```python
from build123d import *

# Parameters (mm, degrees)
F0_R     = 7
F1_DEPTH = 1
F2_R     = 5.5
F3_DEPTH = 8
F4_R     = 7
F5_DEPTH = 7
F6_R     = 0.6
F7_DEPTH = 8
F8_R     = 2.5
F9_DEPTH = 16.001
F10_SIZE = 0.25


with BuildPart() as f1:
    # F0 (on Front) → F1 (new body)
    with BuildSketch(Plane.XZ):
        Circle(F0_R)
    extrude(amount=F1_DEPTH)

    # F2 (on face) → F3 (join)
    with BuildSketch(Plane.XZ.offset(1)):
        Circle(F2_R)
    extrude(amount=F3_DEPTH)

    # F4 (on face) → F5 (join)
    with BuildSketch(Plane.XZ.offset(9)):
        Circle(F4_R)
    extrude(amount=F5_DEPTH)

    # F6 (on face) → F7 (cut, through all)
    with BuildSketch(Plane.XZ.offset(1)):
        with Locations((0, 5.5)):
            Circle(F6_R)
        with Locations((-2.104759, 5.081337)):
            Circle(F6_R)
        with Locations((-3.889087, 3.889087)):
            Circle(F6_R)
        with Locations((-5.081337, 2.104759)):
            Circle(F6_R)
        with Locations((-5.5, 0)):
            Circle(F6_R)
        with Locations((-5.081337, -2.104759)):
            Circle(F6_R)
        with Locations((-3.889087, -3.889087)):
            Circle(F6_R)
        with Locations((-2.104759, -5.081337)):
            Circle(F6_R)
        with Locations((0, -5.5)):
            Circle(F6_R)
        with Locations((2.104759, -5.081337)):
            Circle(F6_R)
        with Locations((3.889087, -3.889087)):
            Circle(F6_R)
        with Locations((5.081337, -2.104759)):
            Circle(F6_R)
        with Locations((5.5, 0)):
            Circle(F6_R)
        with Locations((5.081337, 2.104759)):
            Circle(F6_R)
        with Locations((3.889087, 3.889087)):
            Circle(F6_R)
        with Locations((2.104759, 5.081337)):
            Circle(F6_R)
    extrude(amount=F7_DEPTH, mode=Mode.SUBTRACT)

    # F8 (on face) → F9 (cut, through all)
    with BuildSketch(Plane.XZ.offset(16)):
        Circle(F8_R)
    extrude(amount=-F9_DEPTH, mode=Mode.SUBTRACT)

    # F10
    f10_edges = [f1.edges().sort_by_distance(p)[0] for p in [
        (7, -12.5, 0),
        (-7, -9, 0),
        (-7, -16, 0),
        (7, -0.5, 0),
        (-7, 0, 0),
        (-7, -1, 0),
        (-2.5, -16, 0),
        (2.5, -8, 0),
        (-2.5, 0, 0),
    ]]
    chamfer(f10_edges, length=F10_SIZE)


solid = f1.part
```
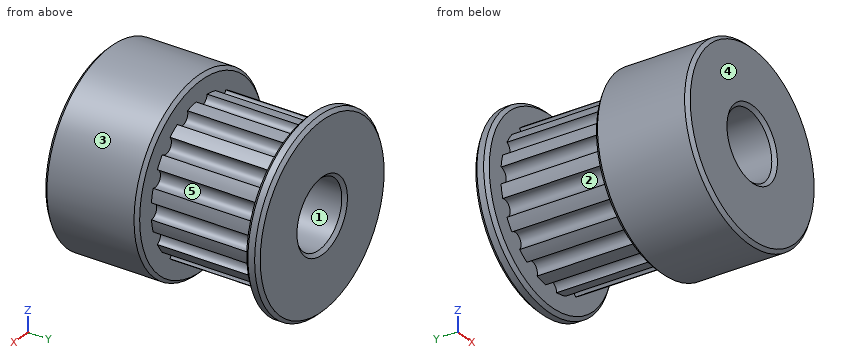
Design review of the part built by this model. Coordinates are the model's own, in mm. Face numbers are marked on the shaded views. A direction names the side the tool comes from. Coordinates: 2 decimals unless noted, no trailing zeros. Loops run counter-clockwise (first coordinate to the right, second up) from the corner with the lowest first, then second, coordinate; pieces in that order, holes last. Notation, with made-up numbers: (3, 81) -> (48, 81) arc R34 ccw to (48, 117) -> close; hole circle Ø4 at (-34.5, -20.5). An arc over 180 degrees is marked (long way). Answer as a JSON object with one key per item and string values.
Q1. Clearance check with a flat-ended pin moving along its axis: pin 1 Ø4 at (x, y) = (1, -6.5) entering from -Z. State where the tip first meets the part, or that it passes through.
Answer block:
{"pin 1": "stops at z = -5.47"}
Q2. The part is to be moulded in two halves that separate along X. For the marked faces 3, 4 and 5, say which applies: +X half, -X half, draft (parallel to the pull), parting line (faces both ways), or undercut.
Answer block:
{"face 3": "parting line", "face 4": "draft", "face 5": "undercut"}
Q3. Take a section at B-B on z = 0. Give the boundary of the cut face in (x, y).
Answer block:
{"outline": "(-7, -15.75) -> (-6.75, -16) -> (-2.75, -16) -> (-2.5, -15.75) -> (-2.5, -0.25) -> (-2.75, 0) -> (-6.75, 0) -> (-7, -0.25) -> (-7, -0.75) -> (-6.75, -1) -> (-4.9, -1) -> (-4.9, -9) -> (-6.75, -9) -> (-7, -9.25) -> close; (2.5, -15.75) -> (2.75, -16) -> (6.75, -16) -> (7, -15.75) -> (7, -9.25) -> (6.75, -9) -> (4.9, -9) -> (4.9, -1) -> (6.75, -1) -> (7, -0.75) -> (7, -0.25) -> (6.75, 0) -> (2.75, 0) -> (2.5, -0.25) -> close"}
Q4. Tool access review of the marked faces 1 and 2: name each direction out of +Z, -Z, +X, -X, +Y, -Y from which nothing blocks a thin tool from reaching the whole face with its end or side.
Answer block:
{"face 1": "+Y, -Y", "face 2": "none"}
Q5. Take a section at A-A on x = 0. Give the boundary of the cut face in (y, z), plus the area to 3 significant figures.
Answer block:
{"outline": "(-16, -6.75) -> (-15.75, -7) -> (-9.25, -7) -> (-9, -6.75) -> (-9, -4.9) -> (-1, -4.9) -> (-1, -6.75) -> (-0.75, -7) -> (-0.25, -7) -> (0, -6.75) -> (0, -2.75) -> (-0.25, -2.5) -> (-15.75, -2.5) -> (-16, -2.75) -> close; (-16, 2.75) -> (-15.75, 2.5) -> (-0.25, 2.5) -> (0, 2.75) -> (0, 6.75) -> (-0.25, 7) -> (-0.75, 7) -> (-1, 6.75) -> (-1, 4.9) -> (-9, 4.9) -> (-9, 6.75) -> (-9.25, 7) -> (-15.75, 7) -> (-16, 6.75) -> close", "area": "110 mm^2"}
Q6. Take a section at D-D on y = -11.25. Give the boundary of the cut face in (x, z).
Answer block:
{"outline": "circle Ø14 at (0, 0); hole circle Ø5 at (0, 0)"}
Q7. To check wall thickness, follow L1, parallel to Y at x = -4, z = -4.25; L2, parallel to Z at x = -5.25, y = -2.5; L3, parallel to X at y = -3.25, z = 4.75. State the ranges of each line that lie inside material, in increasing order.
Answer block:
{"L1": "y = -16 to -9, -1 to 0", "L2": "z = -1.53 to -0.55, 0.55 to 1.53", "L3": "x = -2.77 to -2.6, -1.6 to 1.6, 2.6 to 2.77"}
